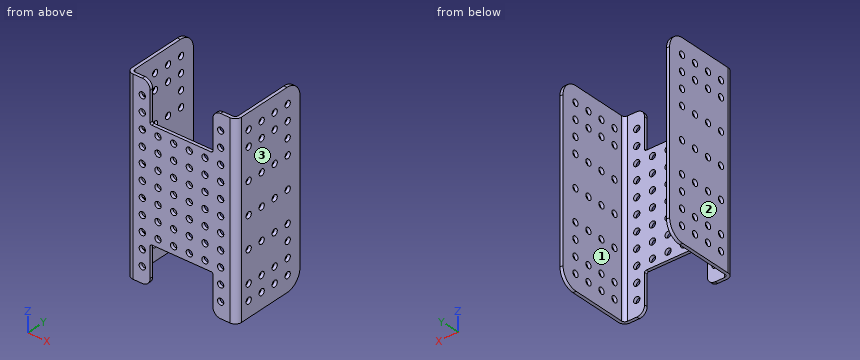
from build123d import *

# Parameters (mm, degrees)
SKETCH1_W                      = 66
SKETCH1_H                      = 120
BOSS_EXTRUDE1_DEPTH            = 2
SKETCH2_R                      = 2
CUT_EXTRUDE1_DEPTH             = 137.967149346
EDGE_FLANGE1_STRIP_W           = 12
EDGE_FLANGE1_STRIP_H           = 2
EDGE_FLANGE1_STRIP_CUT_DEPTH   = 120
EDGE_FLANGE1_STRIP_2_W         = 12
EDGE_FLANGE1_STRIP_2_H         = 2
EDGE_FLANGE1_STRIP_CUT_2_DEPTH = 120
EDGE_FLANGE1_DEPTH             = 120
EDGE_FLANGE1_BEND_DEPTH        = 120
SKETCH24_W                     = 40
SKETCH24_H                     = 25
CUT_EXTRUDE6_DEPTH             = 146.715476186
FILLET1_R                      = 10
FILLET2_R                      = 5
FILLET3_R                      = 1
SKETCH25_R                     = 2
CUT_EXTRUDE8_DEPTH             = 148.312592809


# Sheet-metal steps are written as plain solids
with BuildPart() as part:
    # Sketch1 → Boss-Extrude1 (new body)
    with BuildSketch(Plane(origin=(0, 0, 0), x_dir=(1, 0, 0), z_dir=(0, 1, 0))):
        with Locations((33, 60)):
            Rectangle(SKETCH1_W, SKETCH1_H)
    extrude(amount=BOSS_EXTRUDE1_DEPTH)

    # Sketch2 → Cut-Extrude1 (cut, through all)
    with BuildSketch(Plane(origin=(0, 2, 0), x_dir=(1, 0, 0), z_dir=(0, 1, 0))):
        with Locations(Location((8, 110, 0), (0, 0, 270))):
            Circle(SKETCH2_R)
        with Locations(Location((18, 110, 0), (0, 0, 270))):
            Circle(SKETCH2_R)
        with Locations(Location((28, 110, 0), (0, 0, 270))):
            Circle(SKETCH2_R)
        with Locations(Location((38, 110, 0), (0, 0, 270))):
            Circle(SKETCH2_R)
        with Locations(Location((48, 110, 0), (0, 0, 270))):
            Circle(SKETCH2_R)
        with Locations(Location((58, 110, 0), (0, 0, 270))):
            Circle(SKETCH2_R)
        with Locations(Location((18, 100, 0), (0, 0, 270))):
            Circle(SKETCH2_R)
        with Locations(Location((28, 100, 0), (0, 0, 270))):
            Circle(SKETCH2_R)
        with Locations(Location((38, 100, 0), (0, 0, 270))):
            Circle(SKETCH2_R)
        with Locations(Location((48, 100, 0), (0, 0, 270))):
            Circle(SKETCH2_R)
        with Locations(Location((58, 100, 0), (0, 0, 270))):
            Circle(SKETCH2_R)
        with Locations(Location((18, 90, 0), (0, 0, 270))):
            Circle(SKETCH2_R)
        with Locations(Location((28, 90, 0), (0, 0, 270))):
            Circle(SKETCH2_R)
        with Locations(Location((38, 90, 0), (0, 0, 270))):
            Circle(SKETCH2_R)
        with Locations(Location((48, 90, 0), (0, 0, 270))):
            Circle(SKETCH2_R)
        with Locations(Location((58, 90, 0), (0, 0, 270))):
            Circle(SKETCH2_R)
        with Locations(Location((18, 80, 0), (0, 0, 270))):
            Circle(SKETCH2_R)
        with Locations(Location((28, 80, 0), (0, 0, 270))):
            Circle(SKETCH2_R)
        with Locations(Location((38, 80, 0), (0, 0, 270))):
            Circle(SKETCH2_R)
        with Locations(Location((48, 80, 0), (0, 0, 270))):
            Circle(SKETCH2_R)
        with Locations(Location((58, 80, 0), (0, 0, 270))):
            Circle(SKETCH2_R)
        with Locations(Location((18, 70, 0), (0, 0, 270))):
            Circle(SKETCH2_R)
        with Locations(Location((28, 70, 0), (0, 0, 270))):
            Circle(SKETCH2_R)
        with Locations(Location((38, 70, 0), (0, 0, 270))):
            Circle(SKETCH2_R)
        with Locations(Location((48, 70, 0), (0, 0, 270))):
            Circle(SKETCH2_R)
        with Locations(Location((58, 70, 0), (0, 0, 270))):
            Circle(SKETCH2_R)
        with Locations(Location((18, 60, 0), (0, 0, 270))):
            Circle(SKETCH2_R)
        with Locations(Location((28, 60, 0), (0, 0, 270))):
            Circle(SKETCH2_R)
        with Locations(Location((38, 60, 0), (0, 0, 270))):
            Circle(SKETCH2_R)
        with Locations(Location((48, 60, 0), (0, 0, 270))):
            Circle(SKETCH2_R)
        with Locations(Location((58, 60, 0), (0, 0, 270))):
            Circle(SKETCH2_R)
        with Locations(Location((18, 50, 0), (0, 0, 270))):
            Circle(SKETCH2_R)
        with Locations(Location((28, 50, 0), (0, 0, 270))):
            Circle(SKETCH2_R)
        with Locations(Location((38, 50, 0), (0, 0, 270))):
            Circle(SKETCH2_R)
        with Locations(Location((48, 50, 0), (0, 0, 270))):
            Circle(SKETCH2_R)
        with Locations(Location((58, 50, 0), (0, 0, 270))):
            Circle(SKETCH2_R)
        with Locations(Location((18, 40, 0), (0, 0, 270))):
            Circle(SKETCH2_R)
        with Locations(Location((28, 40, 0), (0, 0, 270))):
            Circle(SKETCH2_R)
        with Locations(Location((38, 40, 0), (0, 0, 270))):
            Circle(SKETCH2_R)
        with Locations(Location((48, 40, 0), (0, 0, 270))):
            Circle(SKETCH2_R)
        with Locations(Location((58, 40, 0), (0, 0, 270))):
            Circle(SKETCH2_R)
        with Locations(Location((18, 30, 0), (0, 0, 270))):
            Circle(SKETCH2_R)
        with Locations(Location((28, 30, 0), (0, 0, 270))):
            Circle(SKETCH2_R)
        with Locations(Location((38, 30, 0), (0, 0, 270))):
            Circle(SKETCH2_R)
        with Locations(Location((48, 30, 0), (0, 0, 270))):
            Circle(SKETCH2_R)
        with Locations(Location((58, 30, 0), (0, 0, 270))):
            Circle(SKETCH2_R)
        with Locations(Location((18, 20, 0), (0, 0, 270))):
            Circle(SKETCH2_R)
        with Locations(Location((28, 20, 0), (0, 0, 270))):
            Circle(SKETCH2_R)
        with Locations(Location((38, 20, 0), (0, 0, 270))):
            Circle(SKETCH2_R)
        with Locations(Location((48, 20, 0), (0, 0, 270))):
            Circle(SKETCH2_R)
        with Locations(Location((58, 20, 0), (0, 0, 270))):
            Circle(SKETCH2_R)
        with Locations(Location((18, 10, 0), (0, 0, 270))):
            Circle(SKETCH2_R)
        with Locations(Location((28, 10, 0), (0, 0, 270))):
            Circle(SKETCH2_R)
        with Locations(Location((38, 10, 0), (0, 0, 270))):
            Circle(SKETCH2_R)
        with Locations(Location((48, 10, 0), (0, 0, 270))):
            Circle(SKETCH2_R)
        with Locations(Location((58, 10, 0), (0, 0, 270))):
            Circle(SKETCH2_R)
        with Locations(Location((8, 100, 0), (0, 0, 270))):
            Circle(SKETCH2_R)
        with Locations(Location((8, 90, 0), (0, 0, 270))):
            Circle(SKETCH2_R)
        with Locations(Location((8, 80, 0), (0, 0, 270))):
            Circle(SKETCH2_R)
        with Locations(Location((8, 70, 0), (0, 0, 270))):
            Circle(SKETCH2_R)
        with Locations(Location((8, 60, 0), (0, 0, 270))):
            Circle(SKETCH2_R)
        with Locations(Location((8, 50, 0), (0, 0, 270))):
            Circle(SKETCH2_R)
        with Locations(Location((8, 40, 0), (0, 0, 270))):
            Circle(SKETCH2_R)
        with Locations(Location((8, 30, 0), (0, 0, 270))):
            Circle(SKETCH2_R)
        with Locations(Location((8, 20, 0), (0, 0, 270))):
            Circle(SKETCH2_R)
        with Locations(Location((8, 10, 0), (0, 0, 270))):
            Circle(SKETCH2_R)
    extrude(amount=-CUT_EXTRUDE1_DEPTH, mode=Mode.SUBTRACT)

    # Edge-Flange1 strip (across the edge) → Edge-Flange1 strip cut (cut)
    with BuildSketch(Plane(origin=(0, 2, -120), x_dir=(1, 0, 0), z_dir=(0, 0, 1))):
        with Locations((-4, -1)):
            Rectangle(EDGE_FLANGE1_STRIP_W, EDGE_FLANGE1_STRIP_H)
    extrude(amount=EDGE_FLANGE1_STRIP_CUT_DEPTH, mode=Mode.SUBTRACT)

    # Edge-Flange1 strip 2 (across the edge) → Edge-Flange1 strip cut 2 (cut)
    with BuildSketch(Plane(origin=(66, 2, 0), x_dir=(-1, 0, 0), z_dir=(0, 0, -1))):
        with Locations((-4, -1)):
            Rectangle(EDGE_FLANGE1_STRIP_2_W, EDGE_FLANGE1_STRIP_2_H)
    extrude(amount=EDGE_FLANGE1_STRIP_CUT_2_DEPTH, mode=Mode.SUBTRACT)

    # Edge-Flange1 section (across the edge) → Edge-Flange1 (add)
    with BuildSketch(Plane(origin=(0, 2, -120), x_dir=(1, 0, 0), z_dir=(0, 0, 1))):
        with BuildLine():
            Line((-2, 2), (-2, 47))
            Line((-2, 47), (0, 47))
            Line((0, 47), (0, 2))
            ThreePointArc((0, 2), (0.585786438, 0.585786438), (2, 0))
            Line((2, 0), (2, -2))
            ThreePointArc((2, -2), (-0.828427125, -0.828427125), (-2, 2))
        make_face()
    extrude(amount=EDGE_FLANGE1_DEPTH)

    # Edge-Flange1 section 2 (across the edge) → Edge-Flange1 bend (add)
    with BuildSketch(Plane(origin=(66, 2, 0), x_dir=(-1, 0, 0), z_dir=(0, 0, -1))):
        with BuildLine():
            Line((-2, 2), (-2, 47))
            Line((-2, 47), (0, 47))
            Line((0, 47), (0, 2))
            ThreePointArc((0, 2), (0.585786438, 0.585786438), (2, 0))
            Line((2, 0), (2, -2))
            ThreePointArc((2, -2), (-0.828427125, -0.828427125), (-2, 2))
        make_face()
    extrude(amount=EDGE_FLANGE1_BEND_DEPTH)

    # Sketch24 → Cut-Extrude6 (cut, through all)
    with BuildSketch(Plane(origin=(0, 2, 0), x_dir=(1, 0, 0), z_dir=(0, 1, 0))):
        with Locations((33, 107.5)):
            Rectangle(SKETCH24_W, SKETCH24_H)
        with Locations((33, 12.5)):
            Rectangle(SKETCH24_W, SKETCH24_H)
    extrude(amount=-CUT_EXTRUDE6_DEPTH, mode=Mode.SUBTRACT)

    # Fillet1
    fillet1_edges = [part.edges().sort_by_distance(p)[0] for p in [
        (-1, 49, -120),
        (-1, 49, 0),
        (67, 49, 0),
        (67, 49, -120),
    ]]
    fillet(fillet1_edges, radius=FILLET1_R)

    # Fillet2
    fillet2_edges = [part.edges().sort_by_distance(p)[0] for p in [
        (13, 1, -120),
        (53, 1, -120),
        (53, 1, 0),
        (13, 1, 0),
    ]]
    fillet(fillet2_edges, radius=FILLET2_R)

    # Fillet3
    fillet3_edges = [part.edges().sort_by_distance(p)[0] for p in [
        (13, 1, -95),
        (53, 1, -95),
        (13, 1, -25),
        (53, 1, -25),
    ]]
    fillet(fillet3_edges, radius=FILLET3_R)

    # Sketch25 → Cut-Extrude8 (cut, through all)
    with BuildSketch(Plane(origin=(68, 0, 0), x_dir=(0, 0, -1), z_dir=(1, 0, 0))):
        with Locations(Location((10, 39.5, 0), (0, 0, 90))):
            Circle(SKETCH25_R)
        with Locations(Location((20, 39.5, 0), (0, 0, 90))):
            Circle(SKETCH25_R)
        with Locations(Location((30, 39.5, 0), (0, 0, 90))):
            Circle(SKETCH25_R)
        with Locations(Location((40, 39.5, 0), (0, 0, 90))):
            Circle(SKETCH25_R)
        with Locations(Location((60, 39.5, 0), (0, 0, 90))):
            Circle(SKETCH25_R)
        with Locations(Location((80, 39.5, 0), (0, 0, 90))):
            Circle(SKETCH25_R)
        with Locations(Location((90, 39.5, 0), (0, 0, 90))):
            Circle(SKETCH25_R)
        with Locations(Location((100, 39.5, 0), (0, 0, 90))):
            Circle(SKETCH25_R)
        with Locations(Location((110, 39.5, 0), (0, 0, 90))):
            Circle(SKETCH25_R)
        with Locations(Location((20, 29.5, 0), (0, 0, 90))):
            Circle(SKETCH25_R)
        with Locations(Location((40, 29.5, 0), (0, 0, 90))):
            Circle(SKETCH25_R)
        with Locations(Location((60, 29.5, 0), (0, 0, 90))):
            Circle(SKETCH25_R)
        with Locations(Location((80, 29.5, 0), (0, 0, 90))):
            Circle(SKETCH25_R)
        with Locations(Location((100, 29.5, 0), (0, 0, 90))):
            Circle(SKETCH25_R)
        with Locations(Location((110, 29.5, 0), (0, 0, 90))):
            Circle(SKETCH25_R)
        with Locations(Location((20, 19.5, 0), (0, 0, 90))):
            Circle(SKETCH25_R)
        with Locations(Location((40, 19.5, 0), (0, 0, 90))):
            Circle(SKETCH25_R)
        with Locations(Location((60, 19.5, 0), (0, 0, 90))):
            Circle(SKETCH25_R)
        with Locations(Location((80, 19.5, 0), (0, 0, 90))):
            Circle(SKETCH25_R)
        with Locations(Location((100, 19.5, 0), (0, 0, 90))):
            Circle(SKETCH25_R)
        with Locations(Location((110, 19.5, 0), (0, 0, 90))):
            Circle(SKETCH25_R)
        with Locations(Location((20, 9.5, 0), (0, 0, 90))):
            Circle(SKETCH25_R)
        with Locations(Location((40, 9.5, 0), (0, 0, 90))):
            Circle(SKETCH25_R)
        with Locations(Location((60, 9.5, 0), (0, 0, 90))):
            Circle(SKETCH25_R)
        with Locations(Location((80, 9.5, 0), (0, 0, 90))):
            Circle(SKETCH25_R)
        with Locations(Location((100, 9.5, 0), (0, 0, 90))):
            Circle(SKETCH25_R)
        with Locations(Location((110, 9.5, 0), (0, 0, 90))):
            Circle(SKETCH25_R)
        with Locations(Location((10, 29.5, 0), (0, 0, 90))):
            Circle(SKETCH25_R)
        with Locations(Location((10, 19.5, 0), (0, 0, 90))):
            Circle(SKETCH25_R)
        with Locations(Location((10, 9.5, 0), (0, 0, 90))):
            Circle(SKETCH25_R)
    extrude(amount=-CUT_EXTRUDE8_DEPTH, mode=Mode.SUBTRACT)


solid = part.part
Work out the finished part from the listing and answer in its coordinate system (mm). Face numbers are marked on the shaded views. Round coordinates to 2 decimals unless told otherwise and drop trailing zeros. Write each loop counter-clockwise with the first axis right and the second up, starting at its lowest first coordinate (ties: lowest second). Pieces come first, ordered by that corner, then holes.
1) Given pin 1 Ø5 at (x, z) = (28, -30) entering from +Y, flat-ended and moving along its own axis, determine where the tip first touches the part or whether it passes through.
2) A cutting plane is placed at D-D (z = -64). Give the vertices of the cut face in (x, y).
3) A cutting plane is placed at C-C (z = -16). Give the vertices of the cut face in (x, y), plus the area to 3 significant figures.
4) A cutting plane is placed at B-B (y = 36). Give the vertices of the cut face in (x, z), plus the area to 3 significant figures.
5) Straight lines are drawn through the part: line 1 (X direction, y = 22, z = -24); line 2 (Y direction, x = 21, z = -74). For each, find the intervals that lie inside material, in ascending order.
6) The mould has two halves that part along X. Classify the marked faces 1, 2 and 3: pulls with the +X half, pulls with the -X half, needs draft (parallel to the pull), parting line crosses it, or undercut.
7) A cutting plane is placed at A-A (x = 48). Give the number of separate pieces and of enclosed holes in the cut face, plus the area to 3 significant figures.
Completed:
1. pin 1: stops at y = 2
2. outline: (-2, 4) arc R4 ccw to (2, 0) - (64, 0) arc R4 ccw to (68, 4) - (68, 49) - (66, 49) - (66, 4) arc R2 cw to (64, 2) - (2, 2) arc R2 cw to (0, 4) - (0, 49) - (-2, 49) - close
3. outline: (-2, 4) arc R4 ccw to (2, 0) - (13, 0) - (13, 2) - (2, 2) arc R2 cw to (0, 4) - (0, 49) - (-2, 49) - close; (53, 0) - (64, 0) arc R4 ccw to (68, 4) - (68, 49) - (66, 49) - (66, 4) arc R2 cw to (64, 2) - (53, 2) - close
3. area: 243 mm2
4. outline: (-2, -120) - (0, -120) - (0, 0) - (-2, 0) - close; (66, -120) - (68, -120) - (68, 0) - (66, 0) - close
4. area: 480 mm2
5. line 1: x = -2 to 0, 66 to 68
5. line 2: y = 0 to 2
6. face 1: undercut
6. face 2: pulls with the -X half
6. face 3: pulls with the +X half
7. separate pieces: 8
7. enclosed holes: 0
7. area: 84.0 mm2
